```python
from build123d import *

# Parameters (mm, degrees)
SKETCH_1_W           = 360
SKETCH_1_H           = 390
EXTRUDE_1_DEPTH      = 23
SKETCH_2_R           = 135
CUT_EXTRUDE_1_DEPTH  = 30
CHAMFER_1_SIZE       = 20
SKETCH_5_R           = 4
CUT_EXTRUDE_2_DEPTH  = 35
SKETCH_6_R           = 7
CUT_EXTRUDE_3_DEPTH  = 35
SKETCH_11_OUTSIDE_W  = 468.25
SKETCH_11_OUTSIDE_H  = 498.25
SKETCH_11_OUTSIDE_R  = 215
CUT_EXTRUDE_8_DEPTH  = 284.776320365
SKETCH_12_R          = 5
CUT_EXTRUDE_9_DEPTH  = 28
SKETCH_13_R          = 5
CUT_EXTRUDE_10_DEPTH = 284.776320365
SKETCH_15_R          = 5
CUT_EXTRUDE_11_DEPTH = 28


with BuildPart() as part:
    # 草图1 → 拉伸1 (new body)
    with BuildSketch(Plane.XY):
        with Locations((-20, 5)):
            Rectangle(SKETCH_1_W, SKETCH_1_H)
    extrude(amount=EXTRUDE_1_DEPTH)

    # 草图2 → 切除-拉伸1 (cut)
    with BuildSketch(Plane.XY.offset(23)):
        with Locations((-20, 5)):
            Circle(SKETCH_2_R)
    extrude(amount=-CUT_EXTRUDE_1_DEPTH, mode=Mode.SUBTRACT)

    # 倒角1
    chamfer_1_edges = [part.edges().sort_by_distance(p)[0] for p in [
        (-200, 200, 11.5),
        (160, 200, 11.5),
        (160, -190, 11.5),
        (-200, -190, 11.5),
    ]]
    chamfer(chamfer_1_edges, length=CHAMFER_1_SIZE)

    # 草图5 → 切除-拉伸2 (cut)
    with BuildSketch(Plane.XY.offset(23)):
        with Locations((52.5, 130.573683549)):
            Circle(SKETCH_5_R)
        with Locations((-20, 150)):
            Circle(SKETCH_5_R)
        with Locations((105.573683549, 77.5)):
            Circle(SKETCH_5_R)
        with Locations((125, 5)):
            Circle(SKETCH_5_R)
        with Locations((105.573683549, -67.5)):
            Circle(SKETCH_5_R)
        with Locations((52.5, -120.573683549)):
            Circle(SKETCH_5_R)
        with Locations((-20, -140)):
            Circle(SKETCH_5_R)
        with Locations((-92.5, -120.573683549)):
            Circle(SKETCH_5_R)
        with Locations((-145.573683549, -67.5)):
            Circle(SKETCH_5_R)
        with Locations((-165, 5)):
            Circle(SKETCH_5_R)
        with Locations((-145.573683549, 77.5)):
            Circle(SKETCH_5_R)
        with Locations((-92.5, 130.573683549)):
            Circle(SKETCH_5_R)
    extrude(amount=-CUT_EXTRUDE_2_DEPTH, mode=Mode.SUBTRACT)

    # 草图6 → 切除-拉伸3 (cut)
    with BuildSketch(Plane.XY.offset(23)):
        with Locations((140, -80)):
            Circle(SKETCH_6_R)
        with Locations((50, 180)):
            Circle(SKETCH_6_R)
        with Locations((140, -155)):
            Circle(SKETCH_6_R)
        with Locations((-90, 180)):
            Circle(SKETCH_6_R)
        with Locations((140, 165)):
            Circle(SKETCH_6_R)
        with Locations((140, 90)):
            Circle(SKETCH_6_R)
        with Locations((50, -170)):
            Circle(SKETCH_6_R)
        with Locations((-90, -170)):
            Circle(SKETCH_6_R)
        with Locations((-180, 90)):
            Circle(SKETCH_6_R)
        with Locations((-180, 165)):
            Circle(SKETCH_6_R)
        with Locations((-180, -155)):
            Circle(SKETCH_6_R)
        with Locations((-180, -80)):
            Circle(SKETCH_6_R)
    extrude(amount=-CUT_EXTRUDE_3_DEPTH, mode=Mode.SUBTRACT)

    # 草图11 outside → 切除-拉伸8 (cut, through all)
    with BuildSketch(Plane.XY.offset(23)):
        with Locations((-20, 5)):
            Rectangle(SKETCH_11_OUTSIDE_W, SKETCH_11_OUTSIDE_H)
        with Locations((-20, 5)):
            Circle(SKETCH_11_OUTSIDE_R, mode=Mode.SUBTRACT)
    extrude(amount=-CUT_EXTRUDE_8_DEPTH, mode=Mode.SUBTRACT)

    # 草图12 → 切除-拉伸9 (cut)
    with BuildSketch(Plane.XY.offset(23)):
        with Locations((-50, 180)):
            Circle(SKETCH_12_R)
        with Locations((10, 180)):
            Circle(SKETCH_12_R)
        with Locations((10, -170)):
            Circle(SKETCH_12_R)
        with Locations((-50, -170)):
            Circle(SKETCH_12_R)
    extrude(amount=-CUT_EXTRUDE_9_DEPTH, mode=Mode.SUBTRACT)

    # 草图13 → 切除-拉伸10 (cut, through all)
    with BuildSketch(Plane.XY.offset(23)):
        with Locations((-20, 180)):
            Circle(SKETCH_13_R)
        with Locations(Location((-20, -170, 0), (0, 0, 180))):
            Circle(SKETCH_13_R)
    extrude(amount=-CUT_EXTRUDE_10_DEPTH, mode=Mode.SUBTRACT)

    # 草图15 → 切除-拉伸11 (cut)
    with BuildSketch(Plane.XY.offset(23)):
        with Locations((-190, 35)):
            Circle(SKETCH_15_R)
        with Locations((150, -25)):
            Circle(SKETCH_15_R)
        with Locations((-190, 5)):
            Circle(SKETCH_15_R)
        with Locations((-190, -25)):
            Circle(SKETCH_15_R)
        with Locations((150, 5)):
            Circle(SKETCH_15_R)
        with Locations((150, 35)):
            Circle(SKETCH_15_R)
    extrude(amount=-CUT_EXTRUDE_11_DEPTH, mode=Mode.SUBTRACT)


solid = part.part
```
Part model, mm, in its own coordinate system. Give positions to 0.01 mm unless a question says otherwise; leave off trailing zeros. Write each loop counter-clockwise with the first axis right and the second up, starting at its lowest first coordinate (ties: lowest second). Pieces come first, ordered by that corner, then holes. Notation, with made-up numbers: (57.5, 27.25) -> (114.5, 27.25) arc R15 cw to (114.5, 47.25) -> close; hole circle Ø1 at (-16.5, -3). An arc over 180 degrees is marked (long way). Put each result on its own line as item: value. Start each with the question number.
Item 1: Cut at C-C (x = 10). List the corners of the cut face in (y, z), then the cut area to 3 significant figures.
Item 2: Pull direction X, two halves, no side cores. Call faces 1 (the face through (134.84, -75.27, 11.66)), 2 (the face through (-161.34, -157.01, 11.66)), 3 (the face through (121.34, 167.01, 11.66)): pulls with the +X half, pulls with the -X half, needs draft (parallel to the pull), parting line crosses it, or undercut.
Item 3: Pin check, flat tip, straight feed: pin 1 Ø8 at (y, z) = (130, 14) entering from +X. Stop position of the tip, or through.
Item 4: Cut at D-D (z = 5.75). State how many separate pieces and enclosed holes the cut face has, then the cut area to 3 significant figures.
Item 5: Cut at B-B (x = 77). List the corners of the cut face in (y, z).
Item 6: Wall check: L1, parallel to Y at x = -20, z = 10.5; L2, parallel to Y at x = 7.5, z = 2.5; L3, parallel to Y at x = -90, z = 11.75. Give the ranges that are in metal, low to high. Write a range as [from, to].
Item 7: Cut at A-A (y = 90). List the corners of the cut face in (x, z), then the cut area to 3 significant figures.
Answer list:
1. outline: (-190, 0) -> (-175, 0) -> (-175, 23) -> (-190, 23) -> close; (-165, 0) -> (-126.62, 0) -> (-126.62, 23) -> (-165, 23) -> close; (136.62, 0) -> (175, 0) -> (175, 23) -> (136.62, 23) -> close; (185, 0) -> (200, 0) -> (200, 23) -> (185, 23) -> close
1. area: 2,460 mm2
2. face 1: undercut
2. face 2: pulls with the -X half
2. face 3: pulls with the +X half
3. pin 1: stops at x = 157.72
4. separate pieces: 1
4. enclosed holes: 33
4. area: 69,100 mm2
5. outline: (-186.87, 0) -> (-88.89, 0) -> (-88.89, 23) -> (-186.87, 23) -> close; (98.89, 0) -> (196.87, 0) -> (196.87, 23) -> (98.89, 23) -> close
6. L1: y = [-190, -175], [-165, -144], [-136, -130], [140, 146], [154, 175], [185, 200]
6. L2: y = [-190, -174.33], [-165.67, -127.17], [137.17, 175.67], [184.33, 200]
6. L3: y = [-190, -177], [-163, -123.7], [-117.45, -110.43], [120.43, 127.45], [133.7, 173], [187, 200]
7. outline: (-200, 0) -> (-187, 0) -> (-187, 23) -> (-200, 23) -> close; (-173, 0) -> (-124.88, 0) -> (-124.88, 23) -> (-173, 23) -> close; (84.88, 0) -> (133, 0) -> (133, 23) -> (84.88, 23) -> close; (147, 0) -> (160, 0) -> (160, 23) -> (147, 23) -> close
7. area: 2,810 mm2
